from build123d import *

# Parameters (mm, degrees)
F2_ANGLE = 106


with BuildPart() as f2:
    # F0 (on Top) → F2 (revolve)
    with BuildSketch(Plane.XY):
        Polygon((5.3707003258, 12), (-5.6292996742, 12), (-5.6292996742, 0), (-2.6292996742, 0), (-2.6292996742, 9), (2.3707003258, 9), (2.3707003258, 0), (5.3707003258, 0), align=None)
    revolve(axis=Axis((0, -132, 0), (1, 0, 0)), revolution_arc=F2_ANGLE)


solid = f2.part
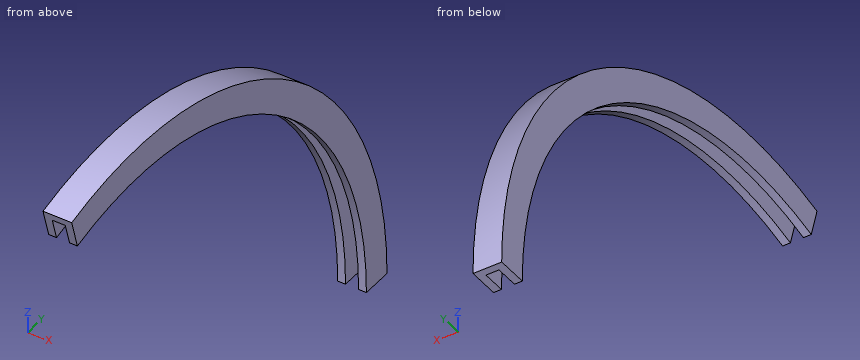
Could you check a few things on this model? Use its own coordinates, in mm. Round coordinates to 2 decimals unless told otherwise and drop trailing zeros. Write each loop counter-clockwise with the first axis right and the second up, starting at its lowest first coordinate (ties: lowest second). Pieces come first, ordered by that corner, then holes. Notation, with made-up numbers: (-35, 19.25) - (-25, 19.25) arc R18 cw to (-25, 44.25) - close; hole circle Ø7 at (-19, 31.25). An arc over 180 degrees is marked (long way). Put each result on its own line as item: value. Start each with the question number.
(1) Will these pins go through, and if not, where does the flat tip stop? pin 1 (6 mm diameter, centred on x = -2, y = -148, fed in from -Z); pin 2 (2 mm diameter, centred on x = 1.5, z = 86.5, fed in from +Y); pin 3 (2 mm diameter, centred on x = 1, z = 20, fed in from -Y).
(2) I want a section at C-C, the plane z = 55. Please give me the cut outline in (x, y).
(3) I want a section at A-A, the plane z = 129. Please give me the cut outline in (x, y).
(4) I need wall thicknesses on probe 1 along X at (y, z) = (-127, 135.5); probe 2 along Y at (x, z) = (-0.5, 53.5); probe 3 along Y at (x, z) = (4, 49.5). Which ranges of each line are inside material? Lowest first, please.
(5) I want a section at B-B, the plane y = -68.5. Please give me the cut outline in (x, z).
(6) I want a section at D-D, the plane x = -0.5. Please give me the cut outline in (y, z), plus the area to 3 significant figures.
Here are the results:
1. pin 1: stops at z = 130.64
1. pin 2: stops at y = -16.13
1. pin 3: stops at y = 7.43
2. outline: (-5.63, -12) - (-2.63, -12) - (-2.63, -2.17) - (2.37, -2.17) - (2.37, -12) - (5.37, -12) - (5.37, 1.08) - (-5.63, 1.08) - close
3. outline: (-5.63, -168.99) - (-2.63, -168.99) - (-2.63, -159.98) - (-5.63, -159.98) - close; (-5.63, -104.02) - (-2.63, -104.02) - (-2.63, -75.08) - (2.37, -75.08) - (2.37, -104.02) - (5.37, -104.02) - (5.37, -68.01) - (-5.63, -68.01) - close; (2.37, -168.99) - (5.37, -168.99) - (5.37, -159.98) - (2.37, -159.98) - close
4. probe 1: x = -5.63 to -2.63, 2.37 to 5.37
4. probe 2: y = -1.54 to 1.69
4. probe 3: y = -9.63 to 3.22
5. outline: (-5.63, 115.72) - (-2.63, 115.72) - (-2.63, 125.89) - (2.37, 125.89) - (2.37, 115.72) - (5.37, 115.72) - (5.37, 129.24) - (-5.63, 129.24) - close
6. outline: (-171.69, 138.42) - (-170.86, 135.54) arc R141 cw to (9, 0) - (12, 0) arc R144 ccw to start
6. area: 791 mm^2
